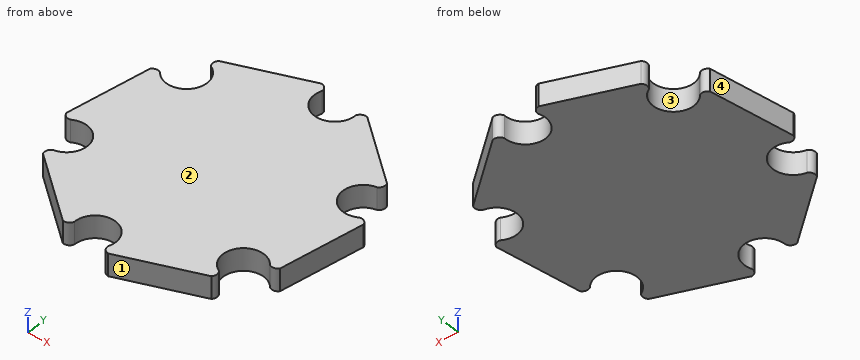
```python
from build123d import *

# Parameters (mm, degrees)
P_IDAT_VYSUNUT_M1_DEPTH = 1.75


with BuildPart() as part:
    # Skica1 → Přidat vysunutím1 (new body)
    with BuildSketch(Plane.XY):
        with BuildLine():
            ThreePointArc((-23.51800991, -0.697818184), (-23.551279529, -0.317829699), (-23.306112267, -0.025612092))
            ThreePointArc((-23.306112267, -0.025612092), (-22.082279375, 2.134290781), (-24.446191601, 2.8924902))
            ThreePointArc((-24.446191601, 2.8924902), (-24.824522171, 2.941112168), (-25.057661359, 3.243013203))
            Line((-25.057661359, 3.243013203), (-24.063340681, 9.771553438))
            ThreePointArc((-24.063340681, 9.771553438), (-23.75089581, 9.990360015), (-23.375244308, 9.924147742))
            ThreePointArc((-23.375244308, 9.924147742), (-20.892797104, 9.944228804), (-21.418133259, 12.370536553))
            ThreePointArc((-21.418133259, 12.370536553), (-21.555999835, 12.731317514), (-21.398375562, 13.083914568))
            Line((-21.398375562, 13.083914568), (-15.289598715, 15.470565049))
            ThreePointArc((-15.289598715, 15.470565049), (-14.935362368, 15.317566791), (-14.79306555, 14.958897763))
            ThreePointArc((-14.79306555, 14.958897763), (-13.534451239, 12.819075952), (-11.695875168, 14.487184282))
            ThreePointArc((-11.695875168, 14.487184282), (-11.443098415, 14.784286161), (-11.054275505, 14.815628758))
            Line((-11.054275505, 14.815628758), (-5.929857109, 10.716094041))
            ThreePointArc((-5.929857109, 10.716094041), (-5.896587491, 10.336105556), (-6.141754752, 10.043887949))
            ThreePointArc((-6.141754752, 10.043887949), (-7.365587644, 7.883985076), (-5.001675418, 7.125785657))
            ThreePointArc((-5.001675418, 7.125785657), (-4.623928538, 7.078562418), (-4.389720717, 6.778446712))
            Line((-4.389720717, 6.778446712), (-5.385684859, 0.239115766))
            ThreePointArc((-5.385684859, 0.239115766), (-5.698895503, 0.026203976), (-6.070920244, 0.097125976))
            ThreePointArc((-6.070920244, 0.097125976), (-8.557586552, 0.076060362), (-8.03228479, -2.354579707))
            ThreePointArc((-8.03228479, -2.354579707), (-7.885616036, -2.705983653), (-8.030385679, -3.058174236))
            Line((-8.030385679, -3.058174236), (-14.178602738, -5.460233693))
            ThreePointArc((-14.178602738, -5.460233693), (-14.524317228, -5.299051786), (-14.654801469, -4.940621906))
            ThreePointArc((-14.654801469, -4.940621906), (-15.913415781, -2.800800095), (-17.751991851, -4.468908425))
            ThreePointArc((-17.751991851, -4.468908425), (-17.989793399, -4.770349614), (-18.371095594, -4.815349636))
            Line((-18.371095594, -4.815349636), (-23.51800991, -0.697818184))
        make_face()
    extrude(amount=P_IDAT_VYSUNUT_M1_DEPTH)


solid = part.part
```
Geometry: final body of the model. Coordinates: model frame, mm. Face numbers are marked on the shaded views. Round coordinates to 2 decimals unless told otherwise and drop trailing zeros. Order: outer loops, then holes, each group sorted by start corner. A loop starts at its lowest first (then second) coordinate and runs counter-clockwise, first axis right, second up. Notation, with made-up numbers: (28, -36.5) -> (87, -36.5) arc R18 cw to (87, -8.5) -> close; hole circle Ø11 at (45.25, 0.25). An arc over 180 degrees is marked (long way). Write each question's results on one line, items separated by ' | '.
Q1. Section query D-D (x = -20). Output: boundary loops of the cut face in (y, z).
Response values:
outline: (-3.51, 0) -> (13.63, 0) -> (13.63, 1.75) -> (-3.51, 1.75) -> close
Q2. Section query B-B (z = 1). Output: boundary loops of the cut face in (x, y), and give its area (3 significant figures).
Response values:
outline: (-25.06, 3.24) arc R0.5 ccw to (-24.45, 2.89) arc R1.6 cw (long way) to (-23.31, -0.03) arc R0.5 ccw to (-23.52, -0.7) -> (-18.37, -4.82) arc R0.5 ccw to (-17.75, -4.47) arc R1.6 cw (long way) to (-14.65, -4.94) arc R0.5 ccw to (-14.18, -5.46) -> (-8.03, -3.06) arc R0.5 ccw to (-8.03, -2.35) arc R1.6 cw (long way) to (-6.07, 0.1) arc R0.49 ccw to (-5.39, 0.24) -> (-4.39, 6.78) arc R0.5 ccw to (-5, 7.13) arc R1.6 cw (long way) to (-6.14, 10.04) arc R0.5 ccw to (-5.93, 10.72) -> (-11.05, 14.82) arc R0.51 ccw to (-11.7, 14.49) arc R1.6 cw (long way) to (-14.79, 14.96) arc R0.5 ccw to (-15.29, 15.47) -> (-21.4, 13.08) arc R0.5 ccw to (-21.42, 12.37) arc R1.6 cw (long way) to (-23.38, 9.92) arc R0.5 ccw to (-24.06, 9.77) -> close | area: 288 mm²
Q3. Pull-direction query (X, two-part tool) for the marked faces 1, 2, 3 and 4; classes: released by +X, released by -X, zero draft, split by the parting line, or undercut.
Response values:
face 1: released by +X | face 2: zero draft | face 3: undercut | face 4: released by -X
Q4. Section query C-C (y = 6). Output: boundary loops of the cut face in (x, z).
Response values:
outline: (-24.64, 0) -> (-4.51, 0) -> (-4.51, 1.75) -> (-24.64, 1.75) -> close
Q5. Pin query (flat end, axial travel): pin 1 Ø1 at (y, z) = (3.5, 1.5) entering from +X; pin 2 Ø5 at (x, y) = (-17.5, 7.5) entering from -Z. Return the tip coordinate at first contact, or that it passes through.
Response values:
pin 1: x = -4.81 | pin 2: z = 0
Q6. Ray query, line 1 along Y through (x, z) = (-23.5, 0.8); line 2 along Y through (x, z) = (-22.25, 0.4); line 3 along X through (y, z) = (3, 0.2). Return the intervals inside material, ascending.
Response values:
line 1: -0.71 to -0.21, 3.15 to 9.98 | line 2: -1.71 to 0.65, 2.45 to 9.35 | line 3: -24.91 to -24.25, -22.89 to -4.97
Q7. Section query A-A (x = -6.75). Output: boundary loops of the cut face in (y, z).
Response values:
outline: (0.58, 0) -> (7.13, 0) -> (7.13, 1.75) -> (0.58, 1.75) -> close; (9.81, 0) -> (11.37, 0) -> (11.37, 1.75) -> (9.81, 1.75) -> close
